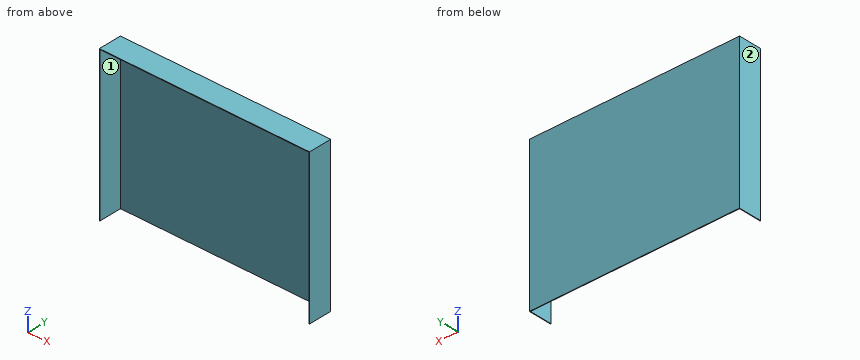
from build123d import *

# Parameters (mm, degrees)
ESBO_O2_W                = 360
ESBO_O2_H                = 260
RESSALTO_EXTRUS_O1_DEPTH = 1
ESBO_O3_W                = 260
ESBO_O3_H                = 40
RESSALTO_EXTRUS_O2_DEPTH = 1
ESBO_O5_W                = 361
ESBO_O5_H                = 40
RESSALTO_EXTRUS_O3_DEPTH = 1
ESBO_O6_W                = 261
ESBO_O6_H                = 40
RESSALTO_EXTRUS_O4_DEPTH = 1


with BuildPart() as part:
    # Esboço2 → Ressalto-extrusão1 (new body)
    with BuildSketch(Plane(origin=(0, 0, 0), x_dir=(1, 0, 0), z_dir=(0, 1, 0))):
        Rectangle(ESBO_O2_W, ESBO_O2_H)
    extrude(amount=RESSALTO_EXTRUS_O1_DEPTH)

    # Esboço3 → Ressalto-extrusão2 (add)
    with BuildSketch(Plane.ZY.offset(180)):
        with Locations((0, -19)):
            Rectangle(ESBO_O3_W, ESBO_O3_H)
    extrude(amount=RESSALTO_EXTRUS_O2_DEPTH)

    # Esboço5 → Ressalto-extrusão3 (add)
    with BuildSketch(Plane.XY.offset(130)):
        with Locations((-0.5, -19)):
            Rectangle(ESBO_O5_W, ESBO_O5_H)
    extrude(amount=RESSALTO_EXTRUS_O3_DEPTH)

    # Esboço6 → Ressalto-extrusão4 (add)
    with BuildSketch(Plane(origin=(180, 0, 0), x_dir=(0, 0, -1), z_dir=(1, 0, 0))):
        with Locations((-0.5, -19)):
            Rectangle(ESBO_O6_W, ESBO_O6_H)
    extrude(amount=RESSALTO_EXTRUS_O4_DEPTH)


solid = part.part
Check sheet for the modelled part. Datum: model origin and axes. Units: mm. Face numbers are marked on the shaded views. A direction names the side the tool comes from. Round coordinates to 2 decimals unless told otherwise and drop trailing zeros. Loops run counter-clockwise (first coordinate to the right, second up) from the corner with the lowest first, then second, coordinate; pieces in that order, holes last. Notation, with made-up numbers: (26.25, -19.5) -> (48.25, -19.5) arc R22 ccw to (48.25, 16.5) -> close; hole circle Ø9 at (-34, -39). An arc over 180 degrees is marked (long way). Put each result on its own line as item: value. Start each with the question number.
1. Section check A-A (y = -13.5). Enter the section's corners in (x, z), plus the area to 3 significant figures.
2. Section check C-C (x = 30). Enter the section's corners in (y, z).
3. Gauge pin test, flat ends, axial feed: pin 1 (1 mm diameter, centred on x = -20.5, z = 40, fed in from -Y); pin 2 (10 mm diameter, centred on x = -69, y = -21.5, fed in from -Z). Record the tip position at first contact, or that the pin passes through.
4. Scan lines: probe 1 along X at (y, z) = (-16, -70.5); probe 2 along Z at (x, y) = (-101.5, -2); probe 3 along Y at (x, z) = (75, -55). Record each from-to range of solid material in increasing order.
5. Section check B-B (z = 87). Enter the section's corners in (x, y).
6. Access from +Z, -Z, +X, -X, +Y, -Y to the whole of each face (thin tool, end or side, straight path). Record for the marked faces 1 and 2.
Findings:
1. outline: (-181, -130) -> (-180, -130) -> (-180, 130) -> (180, 130) -> (180, -130) -> (181, -130) -> (181, 131) -> (-181, 131) -> close
1. area: 882 mm^2
2. outline: (-39, 130) -> (0, 130) -> (0, -130) -> (1, -130) -> (1, 131) -> (-39, 131) -> close
3. pin 1: stops at y = 0
3. pin 2: stops at z = 130
4. probe 1: x = -181 to -180, 180 to 181
4. probe 2: z = 130 to 131
4. probe 3: y = 0 to 1
5. outline: (-181, -39) -> (-180, -39) -> (-180, 0) -> (180, 0) -> (180, -39) -> (181, -39) -> (181, 1) -> (-181, 1) -> close
6. face 1: -Z, -Y
6. face 2: +Z, -Z, -X, +Y, -Y
